Source: three-view drawing plus pictorial views. Frame: mm from the lowest corner of the part. Round coordinates to 2 decimals unless told otherwise and drop trailing zeros. Order: outer loops, then holes, each group sorted by start corner. A loop starts at its lowest first (then second) coordinate and runs counter-clockwise, first axis right, second up. Notation, with made-up numbers: (33, -7) -> (65, -7) arc R24 ccw to (65, 31) -> close; hole circle Ø9 at (27, 85.5). An arc over 180 degrees is marked (long way). Answer as CSV lines item,"result". Start each with the question number.
1) Section query C-C, the plane z = 7. Output: boundary loops of the cut face in (x, y).
2) Line query: L1, parallel to X at y = 17, z = 4.75; L2, parallel to X at y = 18, z = 2.75. Output: solid intervals per line, ascending.
3) First-contact query: P1, Ø4, axis at y = 26.5, z = 8.5, coming from the -X side; P2, Ø6, axis at y = 6.5, z = 5.5, coming from the +X side; P3, Ø1.5, axis at x = 21, y = 27.5, coming from the +Z side. Flat tips, straight axial feed; report the tip coordinate or a pass-through.
4) Mould query, pull axis X, two halves, no side actions, for the marked faces 1, 2 and 3. Classes: +X half, -X half, draft (parallel to the pull), parting line (faces both ways), or undercut.
5) Section query D-D, the plane z = 12.25. Output: boundary loops of the cut face in (x, y), and give its area (3 significant figures).
6) Section query A-A, the plane y = 17. Output: boundary loops of the cut face in (x, z), and give its area (3 significant figures).
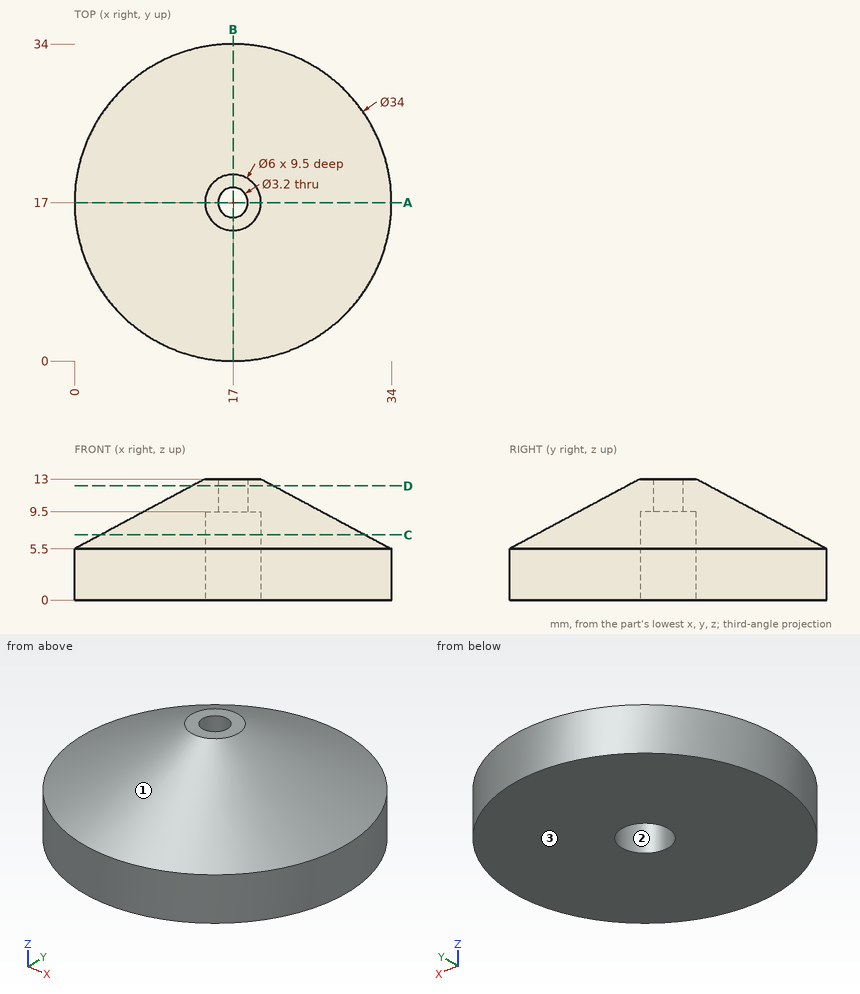
Findings:
1,outline,"circle Ø28.4 at (17, 17); hole circle Ø6 at (17, 17)"
2,L1,"x = 0 to 14, 20 to 34"
2,L2,"x = 0.03 to 14.17, 19.83 to 33.97"
3,P1,"stops at x = 4.97"
3,P2,"stops at x = 32.26"
3,P3,"stops at z = 8.99"
4,face 1,"parting line"
4,face 2,"undercut"
4,face 3,"draft"
5,outline,"circle Ø8.8 at (17, 17); hole circle Ø3.2 at (17, 17)"
5,area,"52.8 mm^2"
6,outline,"(0, 0) -> (14, 0) -> (14, 9.5) -> (15.4, 9.5) -> (15.4, 13) -> (14, 13) -> (0, 5.5) -> close; (18.6, 9.5) -> (20, 9.5) -> (20, 0) -> (34, 0) -> (34, 5.5) -> (20, 13) -> (18.6, 13) -> close"
6,area,"269 mm^2"
